Verification items for the finished model (mm, model axes). A direction names the side the tool comes from. Coordinates: 2 decimals unless noted, no trailing zeros. Return JSON: item names as keys, results as strings.
```python
from build123d import *

# Parameters (mm, degrees)
F3_D     = 6.7564
F3_DEPTH = 5.08
F3_TIP   = 2.0298273432
F7_DEPTH = 0.5
F7_TAPER = 3


with BuildPart() as f1:
    # F0 (on Front) → F1 (revolve)
    with BuildSketch(Plane.XZ):
        with BuildLine():
            Line((-10.7497593308, 0), (0, 0))
            Line((0, 0), (0, 17.3808315196))
            ThreePointArc((0, 17.3808315196), (-0.480802734, 19.7342251413), (-1.8461538462, 21.7104460672))
            ThreePointArc((-1.8461538462, 21.7104460672), (-6.884789629, 25.1797369198), (-12.7647058824, 26.8680539592))
            ThreePointArc((-12.7647058824, 26.8680539592), (-14.3284223283, 26.3770330193), (-15, 24.8819430161))
            ThreePointArc((-15, 24.8819430161), (-14.1991722099, 22.3960149141), (-13.4916369321, 19.8819430161))
            Line((-13.4916369321, 19.8819430161), (-12.9749619928, 19.8819430161))
            ThreePointArc((-12.9749619928, 19.8819430161), (-12.3770619061, 17.3919785968), (-11.8699833059, 14.8819430161))
            Line((-11.8699833059, 14.8819430161), (-12.3783641122, 14.8819430161))
            ThreePointArc((-12.3783641122, 14.8819430161), (-11.9646485976, 12.3885980327), (-11.6412133462, 9.8819430161))
            ThreePointArc((-11.6412133462, 9.8819430161), (-11.2708718222, 4.9478890349), (-11.25, 0))
            Line((-11.25, 0), (-10.7497593308, 0))
        make_face()
        with BuildLine():
            Line((-11.6412133462, 0), (-11.25, 0))
            ThreePointArc((-11.25, 0), (-11.2708718222, 4.9478890349), (-11.6412133462, 9.8819430161))
            Line((-11.6412133462, 9.8819430161), (-11.6412133462, 0))
        make_face()
    revolve(axis=Axis((-7.5, 0, 0), (-1, 0, 0)))

    # F3
    with Locations(Plane.YZ):
        with Locations((0, 0)):
            Hole(F3_D / 2, depth=F3_DEPTH)
            with Locations((0, 0, -(F3_DEPTH + F3_TIP / 2))):  # 118° drill point
                Cone(0, F3_D / 2, F3_TIP, mode=Mode.SUBTRACT)

    # F4 (on face) → F5 (join, up to the next surface of F1)
    with BuildSketch(Plane.YZ):
        with BuildLine():
            Line((-1.190625, 2.187575), (1.190625, 2.187575))
            Line((1.190625, 2.187575), (1.190625, 3.1614312185))
            ThreePointArc((1.190625, 3.1614312185), (0, 3.3782), (-1.190625, 3.1614312185))
            Line((-1.190625, 3.1614312185), (-1.190625, 2.187575))
        make_face()
    extrude(until=Until.NEXT, dir=(-1, 0, 0))

    # F6 (on face) → F7 (cut)
    with BuildSketch(Plane(origin=(-11.6412133462, 0, 0), x_dir=(0, -1, 0), z_dir=(-1, 0, 0))):
        with BuildLine():
            ThreePointArc((9.3982862992, 3.0536883294), (5.8084603689, 7.9946598375), (0, 9.8819430161))
            Line((0, 9.8819430161), (2.2186344386, 3.0536883294))
            Line((2.2186344386, 3.0536883294), (9.3982862992, 3.0536883294))
        make_face()
        with BuildLine():
            Line((-3.5898259303, -1.1664051508), (-9.3982862992, 3.0536883294))
            ThreePointArc((-9.3982862992, 3.0536883294), (-9.3982862992, -3.0536883294), (-5.8084603689, -7.9946598375))
            Line((-5.8084603689, -7.9946598375), (-3.5898259303, -1.1664051508))
        make_face()
        with BuildLine():
            Line((0, -3.7745663573), (-5.8084603689, -7.9946598375))
            ThreePointArc((-5.8084603689, -7.9946598375), (0, -9.8819430161), (5.8084603689, -7.9946598375))
            Line((5.8084603689, -7.9946598375), (0, -3.7745663573))
        make_face()
        with BuildLine():
            ThreePointArc((9.8819430161, 0), (9.7602798995, 1.5458764693), (9.3982862992, 3.0536883294))
            Line((9.3982862992, 3.0536883294), (3.5898259303, -1.1664051508))
            Line((3.5898259303, -1.1664051508), (5.8084603689, -7.9946598375))
            ThreePointArc((5.8084603689, -7.9946598375), (8.804875699, -4.4863082483), (9.8819430161, 0))
        make_face()
        with BuildLine():
            Line((-2.2186344386, 3.0536883294), (0, 9.8819430161))
            ThreePointArc((0, 9.8819430161), (-5.8084603689, 7.9946598375), (-9.3982862992, 3.0536883294))
            Line((-9.3982862992, 3.0536883294), (-2.2186344386, 3.0536883294))
        make_face()
    extrude(amount=-F7_DEPTH, taper=F7_TAPER, mode=Mode.SUBTRACT)


solid = f1.part
```
Q1. Go/stop test with flat-tipped pins: pin 1 (5 mm diameter, centred on y = -8, z = -0.5, fed in from -X); pin 2 (1 mm diameter, centred on x = -2, z = 15, fed in from -Y); pin 3 (8 mm diameter, centred on x = -8, y = -18, fed in from -Z); pin 4 (6 mm diameter, centred on y = 10, z = 13, fed in from +X). Record where each tip stops, or that it passes through.
Values:
{"pin 1": "x = -11.71", "pin 2": "y = -16.66", "pin 3": "z = -21.96", "pin 4": "x = 0"}
Q2. Draft check along Z on faces 1 (the face through (0, -4, 0)), 2 (the face through (-11.141, -1, -7)). Enter one of: pulls with the +Z half, pulls with the -Z half, needs draft (parallel to the pull), parting line crosses it, or undercut.
Values:
{"face 1": "needs draft", "face 2": "undercut"}
Q3. Material ranges on line 1 along Y through (x, z) = (-13.15, 0); line 2 along Y through (x, z) = (-3, 0); line 3 along X through (y, z) = (5.5, 5.5), recorded low to high.
Values:
{"line 1": "-26.88 to -19.88, 19.88 to 26.88", "line 2": "-22.73 to -3.38, 3.38 to 22.73", "line 3": "-11.14 to 0"}
Q4. Tool access check on faces 3 (the face through (-11.141, -4, 6)), 4 (the face through (-3, 0, 2.188)). Record the directions out of +Z, -Z, +X, -X, +Y, -Y that give a thin tool (end or side, any length) a straight path to the whole face; none if there is none.
Values:
{"face 3": "-X", "face 4": "+X"}
